Build history of the part. All positions in model axes, mm. A direction names the side the tool comes from. Give positions to 0.01 mm unless a question says otherwise; leave off trailing zeros. Order: outer loops, then holes, each group sorted by start corner. A loop starts at its lowest first (then second) coordinate and runs counter-clockwise, first axis right, second up. Notation, with made-up numbers: (63.25, 35) - (105.25, 35) arc R18 cw to (105.25, 59) - close; hole circle Ø8 at (-1, -27.75). An arc over 180 degrees is marked (long way). One line per item, written item: value.
```python
from build123d import *

# Parameters (mm, degrees)
F0_W     = 7
F0_H     = 26
F1_DEPTH = 2
F2_START = 10
F2_DEPTH = 2
F3_W     = 7
F3_H     = 12
F4_DEPTH = 2
F5_START = -26
F5_DEPTH = 2
F7_W     = 7
F7_H     = 2
F8_DEPTH = 4
F9_R     = 3.5306


with BuildPart() as f1:
    # F0 (on Front) → F1 (new body)
    with BuildSketch(Plane.XZ):
        with Locations((-3.5, 13)):
            Rectangle(F0_W, F0_H)
    extrude(amount=F1_DEPTH)


with BuildPart() as f2:
    # F0 (on Front) → F2 (new body)
    with BuildSketch(Plane.XZ.offset(F2_START)):
        with Locations((-3.5, 13)):
            Rectangle(F0_W, F0_H)
    extrude(amount=F2_DEPTH)


with BuildPart() as f4:
    # F3 (on face) → F4 (new body)
    with BuildSketch(Plane.XY.offset(26)):
        with Locations((-3.5, -6)):
            Rectangle(F3_W, F3_H)
    extrude(amount=F4_DEPTH)


with BuildPart() as f5:
    # F3 (on face) → F5 (new body)
    with BuildSketch(Plane.XY.offset(26).offset(F5_START)):
        with Locations((-3.5, -6)):
            Rectangle(F3_W, F3_H)
    extrude(amount=-F5_DEPTH)


with BuildPart() as f1_1:
    add(f1.part)

    # F6: union F2, F4, F5
    add(f2.part)
    add(f4.part)
    add(f5.part)

    # F7 (on face) → F8 (cut)
    with BuildSketch(Plane.XZ.offset(12)):
        with Locations((-3.5, 12)):
            Rectangle(F7_W, F7_H)
    extrude(amount=-F8_DEPTH, mode=Mode.SUBTRACT)

    # F9
    f9_edges = [f1_1.edges().sort_by_distance(p)[0] for p in [
        (-3.5, -12, 28),
        (-3.5, 0, 28),
        (-3.5, -12, -2),
        (-3.5, 0, -2),
        (-3.5, -2, 26),
        (-3.5, -2, 0),
        (-3.5, -10, 0),
        (-3.5, -10, 26),
    ]]
    fillet(f9_edges, radius=F9_R)


solid = f1_1.part
```
(1) Slice it at A-A, the plane z = 22. Give the cut face in (x, y).
Completed:
outline: (-7, -12) - (0, -12) - (0, -10) - (-7, -10) - close; (-7, -2) - (0, -2) - (0, 0) - (-7, 0) - close
(2) Slice it at B-B, the plane x = -2.5. Give the cut face in (y, z).
Completed:
outline: (-12, 1.53) arc R3.53 ccw to (-8.47, -2) - (-3.53, -2) arc R3.53 ccw to (0, 1.53) - (0, 24.47) arc R3.53 ccw to (-3.53, 28) - (-8.47, 28) arc R3.53 ccw to (-12, 24.47) - (-12, 13) - (-10, 13) - (-10, 22.47) arc R3.53 cw to (-6.47, 26) - (-5.53, 26) arc R3.53 cw to (-2, 22.47) - (-2, 3.53) arc R3.53 cw to (-5.53, 0) - (-6.47, 0) arc R3.53 cw to (-10, 3.53) - (-10, 11) - (-12, 11) - close
(3) Pin check, flat tips, straight feed: P1, Ø0.6, axis at x = -2, y = -10.5, coming from the -Z side; P2, Ø6, axis at y = -10, z = 19.5, coming from the +X side; P3, Ø2, axis at x = -4, y = -10.5, coming from the +Z side. Stop position of each tip, or through.
Completed:
P1: z = -1.55
P2: x = 0
P3: z = 27.85
(4) 3-axis set-ups, long thin cutter, end or side, ignore diameter. For faces 3 (the face through (-3.45, -8.99, 1.06)), 4 (the face through (-4, -12, 19)), 5 (the face through (-4, -11, 13)): which of +Z, -Z, +X, -X, +Y, -Y reach the whole face in a straight line?
Completed:
face 3: +X, -X
face 4: +Z, -Z, +X, -X, -Y
face 5: +X, -X, -Y
(5) Slice it at C-C, the plane y = -10.5. Give the cut face in (x, z), and give its area (3 significant figures).
Completed:
outline: (-7, -1.36) - (0, -1.36) - (0, 11) - (-7, 11) - close; (-7, 13) - (0, 13) - (0, 27.36) - (-7, 27.36) - close
area: 187 mm²
(6) Pull direction X, two halves, no side cores. Call faces 1 (the face through (-7, -11.4, 13.2)), 2 (the face through (-3.45, -3.06, 1.01)): +X half, -X half, draft (parallel to the pull), parting line (faces both ways), or undercut.
Completed:
face 1: -X half
face 2: draft
(7) Drill centre lines: line 1 (Y direction, x = -4.75, z = 20); line 2 (Y direction, x = -3.75, z = 12.25); line 3 (Z direction, x = -2.75, y = -9.5). Where is each one in solid material? Low to high.
Completed:
line 1: -12 to -10, -2 to 0
line 2: -2 to 0
line 3: -1.85 to 1.72, 24.28 to 27.85
